Can you work these out from the model? Positions are in its coordinate system, mm. Face numbers are marked on the shaded views. A direction names the side the tool comes from. Coordinates: 2 decimals unless noted, no trailing zeros. Order: outer loops, then holes, each group sorted by start corner. A loop starts at its lowest first (then second) coordinate and runs counter-clockwise, first axis right, second up. Notation, with made-up numbers: (43.25, 50.5) -> (49.25, 50.5) arc R26 cw to (49.25, 81.5) -> close; hole circle Ø5 at (38.25, 4.25). An arc over 180 degrees is marked (long way). Use a Markdown table: item, result. Add a question column.
1. If I drill on line 1 along X through (y, z) = (-1.5, 1.95); line 2 along Y through (x, z) = (0, 0.7); line 3 along Y through (x, z) = (30.75, 1.45), over which ranges is the centre line in solid material (lowest first)? Write a range as from..to.
2. For pin 1 Ø1 at (x, z) = (19.5, 1.5) entering from -Y; pin 2 Ø1.5 at (y, z) = (-6.5, 2) entering from +X, each with a flat end and sliding along its axis, tell me the tip position at first contact or that it passes through.
3. Suppose I cut it at B-B, the plane y = -8.75. List the corners of the cut face in (x, z) for me.
4. We'd pull the mould along X, two halves only. Please class the marked faces 1, 2 and 3: pulls with the +X half, pulls with the -X half, needs draft (parallel to the pull), parting line crosses it, or undercut.
5. For the marked faces 4, 5 and 6, which set-ups out of +Z, -Z, +X, -X, +Y, -Y let a thin tool reach every point of the face, with its end or its side?
6. Suppose I cut it at A-A, the plane z = 1.5. State how many separate pieces and enclosed holes the cut face has, then the cut area to 3 significant figures.
```python
from build123d import *

# Parameters (mm, degrees)
SKETCH1_R           = 1.75
BOSS_EXTRUDE1_DEPTH = 3.5
SKETCH2_R           = 3
CUT_EXTRUDE1_DEPTH  = 38.866203929


with BuildPart() as part:
    # Sketch1 → Boss-Extrude1 (new body)
    with BuildSketch(Plane.XY):
        with BuildLine():
            Line((0.31, 14.63), (-0.31, 14.63))
            ThreePointArc((-0.31, 14.63), (-0.838273314, 13.383704325), (-1.04, 12.04518576))
            ThreePointArc((-1.04, 12.04518576), (-1.578061664, 11.986568374), (-2.112960617, 11.903927815))
            ThreePointArc((-2.112960617, 11.903927815), (-2.65424773, 13.144626757), (-3.487085624, 14.211728743))
            Line((-3.487085624, 14.211728743), (-4.085959636, 14.051260935))
            ThreePointArc((-4.085959636, 14.051260935), (-4.273667417, 12.71070456), (-4.122086336, 11.365584201))
            ThreePointArc((-4.122086336, 11.365584201), (-4.626642697, 11.169703548), (-5.12192646, 10.951436862))
            ThreePointArc((-5.12192646, 10.951436862), (-5.965886177, 12.009764599), (-7.046532125, 12.824951657))
            Line((-7.046532125, 12.824951657), (-7.583467875, 12.514951657))
            ThreePointArc((-7.583467875, 12.514951657), (-7.417818147, 11.171491285), (-6.9232593, 9.911436862))
            ThreePointArc((-6.9232593, 9.911436862), (-7.359925677, 9.591641884), (-7.781841479, 9.252623584))
            ThreePointArc((-7.781841479, 9.252623584), (-8.870959341, 10.05645683), (-10.125769107, 10.564175311))
            Line((-10.125769107, 10.564175311), (-10.564175311, 10.125769107))
            ThreePointArc((-10.564175311, 10.125769107), (-10.05645683, 8.870959341), (-9.252623584, 7.781841479))
            ThreePointArc((-9.252623584, 7.781841479), (-9.591641884, 7.359925677), (-9.911436862, 6.9232593))
            ThreePointArc((-9.911436862, 6.9232593), (-11.171491285, 7.417818147), (-12.514951657, 7.583467875))
            Line((-12.514951657, 7.583467875), (-12.824951657, 7.046532125))
            ThreePointArc((-12.824951657, 7.046532125), (-12.009764599, 5.965886177), (-10.951436862, 5.12192646))
            ThreePointArc((-10.951436862, 5.12192646), (-11.169703548, 4.626642697), (-11.365584201, 4.122086336))
            ThreePointArc((-11.365584201, 4.122086336), (-12.71070456, 4.273667417), (-14.051260935, 4.085959636))
            Line((-14.051260935, 4.085959636), (-14.211728743, 3.487085624))
            ThreePointArc((-14.211728743, 3.487085624), (-13.144626757, 2.65424773), (-11.903927815, 2.112960617))
            ThreePointArc((-11.903927815, 2.112960617), (-11.986568374, 1.578061664), (-12.04518576, 1.04))
            ThreePointArc((-12.04518576, 1.04), (-13.383704325, 0.838273314), (-14.63, 0.31))
            Line((-14.63, 0.31), (-14.63, -0.31))
            ThreePointArc((-14.63, -0.31), (-13.383704325, -0.838273314), (-12.04518576, -1.04))
            ThreePointArc((-12.04518576, -1.04), (-11.986568374, -1.578061664), (-11.903927815, -2.112960617))
            ThreePointArc((-11.903927815, -2.112960617), (-13.144626757, -2.65424773), (-14.211728743, -3.487085624))
            Line((-14.211728743, -3.487085624), (-14.051260935, -4.085959636))
            ThreePointArc((-14.051260935, -4.085959636), (-12.71070456, -4.273667417), (-11.365584201, -4.122086336))
            ThreePointArc((-11.365584201, -4.122086336), (0.064808849, -12.089826294), (11.409123542, -4))
            Line((11.409123542, -4), (30.75, -4))
            ThreePointArc((30.75, -4), (34.75, 0), (30.75, 4))
            Line((30.75, 4), (11.409123542, 4))
            ThreePointArc((11.409123542, 4), (11.194344337, 4.566700654), (10.951436862, 5.12192646))
            ThreePointArc((10.951436862, 5.12192646), (12.009764599, 5.965886177), (12.824951657, 7.046532125))
            Line((12.824951657, 7.046532125), (12.514951657, 7.583467875))
            ThreePointArc((12.514951657, 7.583467875), (11.171491285, 7.417818147), (9.911436862, 6.9232593))
            ThreePointArc((9.911436862, 6.9232593), (9.591641884, 7.359925677), (9.252623584, 7.781841479))
            ThreePointArc((9.252623584, 7.781841479), (10.05645683, 8.870959341), (10.564175311, 10.125769107))
            Line((10.564175311, 10.125769107), (10.125769107, 10.564175311))
            ThreePointArc((10.125769107, 10.564175311), (8.870959341, 10.05645683), (7.781841479, 9.252623584))
            ThreePointArc((7.781841479, 9.252623584), (7.359925677, 9.591641884), (6.9232593, 9.911436862))
            ThreePointArc((6.9232593, 9.911436862), (7.417818147, 11.171491285), (7.583467875, 12.514951657))
            Line((7.583467875, 12.514951657), (7.046532125, 12.824951657))
            ThreePointArc((7.046532125, 12.824951657), (5.965886177, 12.009764599), (5.12192646, 10.951436862))
            ThreePointArc((5.12192646, 10.951436862), (4.626642697, 11.169703548), (4.122086336, 11.365584201))
            ThreePointArc((4.122086336, 11.365584201), (4.273667417, 12.71070456), (4.085959636, 14.051260935))
            Line((4.085959636, 14.051260935), (3.487085624, 14.211728743))
            ThreePointArc((3.487085624, 14.211728743), (2.65424773, 13.144626757), (2.112960617, 11.903927815))
            ThreePointArc((2.112960617, 11.903927815), (1.578061664, 11.986568374), (1.04, 12.04518576))
            ThreePointArc((1.04, 12.04518576), (0.838273314, 13.383704325), (0.31, 14.63))
        make_face()
        with Locations((30.75, 0)):
            Circle(SKETCH1_R, mode=Mode.SUBTRACT)
        Circle(SKETCH1_R, mode=Mode.SUBTRACT)
    extrude(amount=BOSS_EXTRUDE1_DEPTH)

    # Sketch2 → Cut-Extrude1 (cut, through all)
    with BuildSketch(Plane.XY.offset(3.5)):
        Circle(SKETCH2_R)
    extrude(amount=-CUT_EXTRUDE1_DEPTH, mode=Mode.SUBTRACT)


solid = part.part
```
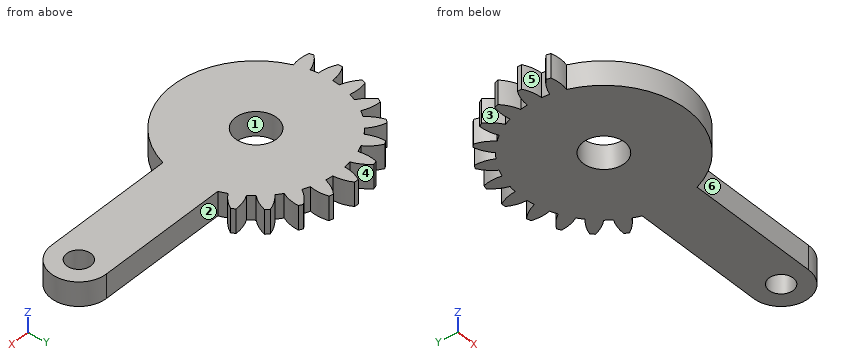
Worked out:
| question | item | result |
|---|---|---|
| 1 | line 1 | x = -12..-2.6, 2.6..29.85, 31.65..34.46 |
| 1 | line 2 | y = -12.09..-3, 3..14.63 |
| 1 | line 3 | y = -4..-1.75, 1.75..4 |
| 2 | pin 1 | stops at y = -4 |
| 2 | pin 2 | stops at x = 10.64 |
| 3 | outline | (-8.34, 0) -> (8.34, 0) -> (8.34, 3.5) -> (-8.34, 3.5) -> close |
| 4 | face 1 | undercut |
| 4 | face 2 | needs draft |
| 4 | face 3 | pulls with the -X half |
| 5 | face 4 | +Z, -Z, +Y |
| 5 | face 5 | +Z, -Z, -X |
| 5 | face 6 | +Z, -Z, +X, -Y |
| 6 | separate pieces | 1 |
| 6 | enclosed holes | 2 |
| 6 | area | 646 mm² |
